Source: CAD feature listing. Evaluate the final solid. Frame: model axes, mm. Give positions to 0.01 mm unless a question says otherwise; leave off trailing zeros. Loops run counter-clockwise (first coordinate to the right, second up) from the corner with the lowest first, then second, coordinate; pieces in that order, holes last. Notation, with made-up numbers: (57.5, 63) -> (90.5, 63) arc R34 cw to (90.5, 94) -> close; hole circle Ø1 at (-31.5, 54.5). An arc over 180 degrees is marked (long way). Answer as a JSON object with one key per item and string values. Group by question number.
from build123d import *

# Parameters (mm, degrees)
SKETCH2_R           = 3.175
BOSS_EXTRUDE1_DEPTH = 3.175


with BuildPart() as part:
    # Sketch2 → Boss-Extrude1 (new, symmetric)
    with BuildSketch(Plane(origin=(0, 0, 0), x_dir=(1, 0, 0), z_dir=(0, 1, 0))):
        with BuildLine():
            ThreePointArc((-19.05, -20.32), (-17.562102448, -23.912102448), (-13.97, -25.4))
            Line((-13.97, -25.4), (13.97, -25.4))
            ThreePointArc((13.97, -25.4), (17.562102448, -23.912102448), (19.05, -20.32))
            Line((19.05, -20.32), (19.05, 25.4))
            ThreePointArc((19.05, 25.4), (0, 27.773915087), (-19.05, 25.4))
            Line((-19.05, 25.4), (-19.05, -20.32))
        make_face()
        with Locations(Location((0, -19.05, 0), (0, 0, 270))):
            Circle(SKETCH2_R, mode=Mode.SUBTRACT)
    extrude(amount=BOSS_EXTRUDE1_DEPTH, both=True)


solid = part.part
(1) Mould query, pull axis Z, two halves, no side actions, for faces 1 (the face through (0.14, -0.04, 15.88)), 2 (the face through (17.522, 0.044, 23.951)), 3 (the face through (0.269, 0.044, -27.773)). Classes: pulls with the +Z half, pulls with the -Z half, needs draft (parallel to the pull), parting line crosses it, or undercut.
(2) Section query B-B on z = 19.05. Return the cut outline in (x, y) (3 decimals).
(3) Material intervals for line 1 (X direction, y = 0.75, z = 19.05) (3 decimals); line 2 (Z direction, x = -16.5, y = -3); line 3 (Z direction, x = 6, y = 2.5), sorted ascending. Write a range as from..to.
(4) Section query D-D on x = -15.5. Return the cut outline in (y, z) (3 decimals), plus the area to 3 significant figures.
(5) Section query A-A on x = 0. Return the cut outline in (y, z) (3 decimals), plus the area to 3 significant figures.
(6) Section query C-C on y = 1.75. Return the cut outline in (x, z) (3 decimals), plus the area to 3 significant figures.
Result:
{
 "1": {"face 1": "undercut", "face 2": "pulls with the +Z half", "face 3": "pulls with the -Z half"},
 "2": {"outline": "(-19.05, -3.175) -> (-3.175, -3.175) -> (-3.175, 3.175) -> (-19.05, 3.175) -> close; (3.175, -3.175) -> (19.05, -3.175) -> (19.05, 3.175) -> (3.175, 3.175) -> close"},
 "3": {"line 1": "-19.05..-3.175, 3.175..19.05", "line 2": "-26..24.73", "line 3": "-27.54..25.4"},
 "4": {"outline": "(-3.175, -26.211) -> (3.175, -26.211) -> (3.175, 25.164) -> (-3.175, 25.164) -> close", "area": "326 mm²"},
 "5": {"outline": "(-3.175, -27.774) -> (3.175, -27.774) -> (3.175, 15.875) -> (-3.175, 15.875) -> close; (-3.175, 22.225) -> (3.175, 22.225) -> (3.175, 25.4) -> (-3.175, 25.4) -> close", "area": "297 mm²"},
 "6": {"outline": "(-19.05, -25.4) arc R77.622 ccw to (19.05, -25.4) -> (19.05, 20.32) arc R5.08 ccw to (13.97, 25.4) -> (-13.97, 25.4) arc R5.08 ccw to (-19.05, 20.32) -> close; hole circle Ø6.35 at (0, 19.05)", "area": "1,950 mm²"}
}
